Geometry check sheet. Reference: the model listing, model coordinates, mm. A direction names the side the tool comes from. Round coordinates to 2 decimals unless told otherwise and drop trailing zeros. Loops run counter-clockwise (first coordinate to the right, second up) from the corner with the lowest first, then second, coordinate; pieces in that order, holes last. Notation, with made-up numbers: (26.5, 34.25) - (78.5, 34.25) arc R26 cw to (78.5, 57.25) - close; hole circle Ø3 at (14, -39). An arc over 180 degrees is marked (long way). Answer in a Markdown table with one row per item. Add a question column.
```python
from build123d import *

# Parameters (mm, degrees)
SKETCH1_W          = 63.5
SKETCH1_H          = 50.8
EXTRUDE1_DEPTH     = 82.423
SKETCH5_R          = 22.225
EXTRUDE2_DEPTH     = 5.969
SKETCH6_W          = 14.2875
SKETCH6_H          = 29.083
CUT_EXTRUDE4_DEPTH = 30.48
HOLE1_D            = 8.7376
HOLE1_DEPTH        = 82.423
HOLE2_D            = 8.7376
HOLE2_DEPTH        = 50.8
LPATTERN1_COUNT    = 2
LPATTERN1_PITCH    = 25.4


with BuildPart() as part:
    # Sketch1 → Extrude1 (new body)
    with BuildSketch(Plane(origin=(0, 0, 0), x_dir=(0, 0, -1), z_dir=(1, 0, 0))):
        Rectangle(SKETCH1_W, SKETCH1_H)
    extrude(amount=EXTRUDE1_DEPTH)

    # S2D0002 → Cut-Revolve1 (revolve, cut)
    with BuildSketch(Plane(origin=(0, 17.4498, 0), x_dir=(-1, 0, 0), z_dir=(0, 1, 0)), mode=Mode.PRIVATE) as cut_revolve1_sk:
        Polygon((-18.8849, -31.496), (-22.225, -31.496), (-22.225, -31.75), (-12.7, -31.75), (-12.7, -17.526), (-17.6784, -17.526), (-17.6784, -28.279393135), (-18.342306865, -28.9433), align=None)
    revolve(cut_revolve1_sk.sketch.rotate(Axis((12.7, 17.4498, -19.13842003), (0, 0, 1)), 180), axis=Axis((12.7, 17.4498, -19.13842003), (0, 0, 1)), mode=Mode.SUBTRACT)  # turned: the seam where the file's is

    # Sketch3 → Cut-Revolve2 (revolve, cut)
    with BuildSketch(Plane(origin=(41.148, 0, -25.146), x_dir=(1, 0, 0), z_dir=(0, 1, 0))):
        Polygon((31.5849, 6.35), (34.925, 6.35), (34.925, 6.604), (25.4, 6.604), (25.4, -7.62), (30.3784, -7.62), (30.3784, 3.133393135), (31.042306865, 3.7973), align=None)
    revolve(axis=Axis((66.548, 0, -3.189624441), (0, 0, -1)), mode=Mode.SUBTRACT)

    # Sketch4 → Cut-Revolve3 (revolve, cut)
    with BuildSketch(Plane(origin=(53.975, 0, 0), x_dir=(0, -1, 0), z_dir=(0, 0, 1)), mode=Mode.PRIVATE) as cut_revolve3_sk:
        Polygon((6.1849, 25.4), (9.525, 25.4), (9.525, 28.448), (0, 28.448), (0, 14.0462), (4.9784, 14.0462), (4.9784, 22.183393135), (5.642306865, 22.8473), align=None)
    revolve(cut_revolve3_sk.sketch.rotate(Axis((38.879609832, 0, 0), (1, 0, 0)), 270), axis=Axis((38.879609832, 0, 0), (1, 0, 0)), mode=Mode.SUBTRACT)  # turned: the seam where the file's is

    # Sketch5 → Extrude2 (add)
    with BuildSketch(Plane.ZY):
        Circle(SKETCH5_R)
    extrude(amount=EXTRUDE2_DEPTH)

    # Sketch6 → Revolve1 (revolve)
    with BuildSketch(Plane(origin=(0, 0, 0), x_dir=(0, 0, 1), z_dir=(0, -1, 0)), mode=Mode.PRIVATE) as revolve1_sk:
        with Locations((-7.14375, 20.5105)):
            Rectangle(SKETCH6_W, SKETCH6_H)
    revolve(revolve1_sk.sketch.rotate(Axis((5.754582971, 0, 0), (-1, 0, 0)), 180), axis=Axis((5.754582971, 0, 0), (-1, 0, 0)))  # turned: the seam where the file's is

    # S2D0001 → Cut-Revolve4 (revolve, cut)
    with BuildSketch(Plane(origin=(-18.511260017, 3.2639, 0), x_dir=(0, 1, 0), z_dir=(0, 0, 1)), mode=Mode.PRIVATE) as cut_revolve4_sk:
        Polygon((2.286, 14.473017728), (2.286, -1.950460017), (-3.2639, -1.950460017), (-3.2639, 16.540739983), (3.4798, 16.540739983), align=None)
    revolve(cut_revolve4_sk.sketch.rotate(Axis((0, 0, 0), (-1, 0, 0)), 270), axis=Axis((0, 0, 0), (-1, 0, 0)), mode=Mode.SUBTRACT)  # turned: the seam where the file's is

    # Sketch8 → Cut-Revolve5 (revolve, cut)
    with BuildSketch(Plane(origin=(0, 0, 0), x_dir=(0, 0, -1), z_dir=(0, 1, 0)), mode=Mode.PRIVATE) as cut_revolve5_sk:
        with BuildLine():
            Line((-14.2875, 25.146), (-14.097, 25.908))
            Line((-14.097, 25.908), (-14.097, 34.036))
            ThreePointArc((-14.097, 34.036), (-13.996678675, 34.579796865), (-13.708922533, 35.052))
            Line((-13.708922533, 35.052), (-14.2875, 35.052))
            Line((-14.2875, 35.052), (-14.2875, 25.146))
        make_face()
    revolve(cut_revolve5_sk.sketch.rotate(Axis((-12.65936, 0, 0), (-1, 0, 0)), 180), axis=Axis((-12.65936, 0, 0), (-1, 0, 0)), mode=Mode.SUBTRACT)  # turned: the seam where the file's is

    # Sketch12 → Cut-Extrude4 (cut, symmetric)
    with BuildSketch(Plane(origin=(0, 0, 0), x_dir=(0, -1, 0), z_dir=(0, 0, -1))):
        Polygon((12.573, 35.052), (12.573, 27.4828), (14.097, 25.9588), (14.097, 35.052), align=None)
        Polygon((-12.573, 35.052), (-12.573, 27.4828), (-14.097, 25.9588), (-14.097, 35.052), align=None)
    extrude(amount=CUT_EXTRUDE4_DEPTH, both=True, mode=Mode.SUBTRACT)

    # Hole1
    with Locations(Plane.ZY):
        with Locations((-24.13, -17.78), (24.13, 17.78)):
            Hole(HOLE1_D / 2, depth=HOLE1_DEPTH)

    # Hole2
    with Locations(Plane(origin=(0, 25.4, 0), x_dir=(-1, 0, 0), z_dir=(0, 1, 0))):
        with Locations((-26.797, -25.4), (-26.797, 25.4)):
            hole2 = Hole(HOLE2_D / 2, depth=HOLE2_DEPTH)

    # LPattern1: Hole2 ×2
    with Locations(*[(i * LPATTERN1_PITCH, 0, 0) for i in range(1, LPATTERN1_COUNT)]):
        add(hole2, mode=Mode.SUBTRACT)


solid = part.part
```
Q1. Depth check by flat-ended pin: P1, Ø2, axis at y = 10, z = -22, coming from the -X side; P2, Ø6, axis at y = 0, z = 0, coming from the +X side; P3, Ø2, axis at y = 19.5, z = 11.5, coming from the -X side. Enter the tip coordinate at first touch or a pass-through.
Q2. Scan lines: line 1 (X direction, y = -1, z = 25); line 2 (Y direction, x = 17.5, z = 24.5); line 3 (X direction, y = 17.5, z = -27.5). Record each from-to range of solid material in increasing order. Write a range as from..to.
Q3. Cross-section at D-D, the plane y = 0. State how many separate pieces and enclosed holes the cut face has, plus the area to 3 significant figures.
Q4. Release check for a two-part mould opening along Z. For faces 1 (the flat face through (0, 6, 22)), 2 (the flat face through (41, 0, -31.75)), 3 (the cylindrical face through (41.788, -17.588, -19.765)) record: +Z half, -Z half, draft (parallel to the pull), parting line (faces both ways), or undercut.
Q5. Cross-section at A-A, the plane y = -17.78. Enter the section's corners in (x, z) (3 decimals), plus the area to 3 significant figures.
Q6. Set-up check for faces 4 (the flat face through (41, -25.4, 0)), 5 (the flat face through (67, 0, -17.526)), 6 (the cylindrical face through (-30.029, -4.234, -13.446)): record each of +Z, -Z, +X, -X, +Y, -Y from which the full face is reachable in a straight line by a thin tool's end or side.
Q7. Cross-section at B-B, the plane z = -24.13. Enter the section's corners in (x, y), plus the area to 3 significant figures.
Q8. Cross-section at C-C, the plane z = 24.13. Enter the section's corners in (x, y).
Check sheet entries:
| question | item | result |
|---|---|---|
| 1 | P1 | x = 0 |
| 1 | P2 | x = 68.02 |
| 1 | P3 | x = -5.97 |
| 2 | line 1 | 0..22.45, 31.15..47.85, 56.55..82.42 |
| 2 | line 2 | -25.4..13.43, 22.13..25.4 |
| 2 | line 3 | 0..7.72, 17.68..22.97, 30.63..48.37, 56.03..82.42 |
| 3 | separate pieces | 1 |
| 3 | enclosed holes | 4 |
| 3 | area | 5,550 mm² |
| 4 | face 1 | draft |
| 4 | face 2 | -Z half |
| 4 | face 3 | undercut |
| 5 | outline | (-5.969, -13.335) - (0, -13.335) - (0, -19.761) - (82.423, -19.761) - (82.423, 31.75) - (0, 31.75) - (0, 13.335) - (-5.969, 13.335) - close; (0, -31.75) - (82.423, -31.75) - (82.423, -28.499) - (55.277, -28.499) arc R4.369 cw to (49.117, -28.499) - (29.877, -28.499) arc R4.369 cw to (23.717, -28.499) - (0, -28.499) - close; hole circle Ø8.738 at (26.797, 25.4); hole circle Ø8.738 at (52.197, 25.4) |
| 5 | area | 4,540 mm² |
| 6 | face 4 | +Z, -Z, +X, -X, -Y |
| 6 | face 5 | -Z |
| 6 | face 6 | -X |
| 7 | outline | (0, -25.4) - (22.62, -25.4) - (22.62, -22.15) - (0, -22.15) - close; (0, -13.41) - (22.62, -13.41) - (22.62, 25.4) - (0, 25.4) - close; (30.98, -25.4) - (48.02, -25.4) - (48.02, -22.15) - (30.98, -22.15) - close; (30.98, -13.41) - (48.02, -13.41) - (48.02, 25.4) - (30.98, 25.4) - close; (56.38, -25.4) - (82.42, -25.4) - (82.42, -22.15) - (56.38, -22.15) - close; (56.38, -13.41) - (82.42, -13.41) - (82.42, 25.4) - (56.38, 25.4) - close; hole circle Ø9.96 at (12.7, 17.45); hole circle Ø9.96 at (66.55, 0) |
| 7 | area | 2,610 mm² |
| 8 | outline | (0, -25.4) - (22.62, -25.4) - (22.62, 13.41) - (0, 13.41) - close; (0, 22.15) - (22.62, 22.15) - (22.62, 25.4) - (0, 25.4) - close; (30.98, -25.4) - (48.02, -25.4) - (48.02, 13.41) - (30.98, 13.41) - close; (30.98, 22.15) - (48.02, 22.15) - (48.02, 25.4) - (30.98, 25.4) - close; (56.38, -25.4) - (82.42, -25.4) - (82.42, 13.41) - (56.38, 13.41) - close; (56.38, 22.15) - (82.42, 22.15) - (82.42, 25.4) - (56.38, 25.4) - close |
